For this review, take the finished solid that the model builds, in its own axes (mm). Face numbers are marked on the shaded views. A direction names the side the tool comes from. Coordinates: 2 decimals unless noted, no trailing zeros. Order: outer loops, then holes, each group sorted by start corner. A loop starts at its lowest first (then second) coordinate and runs counter-clockwise, first axis right, second up.
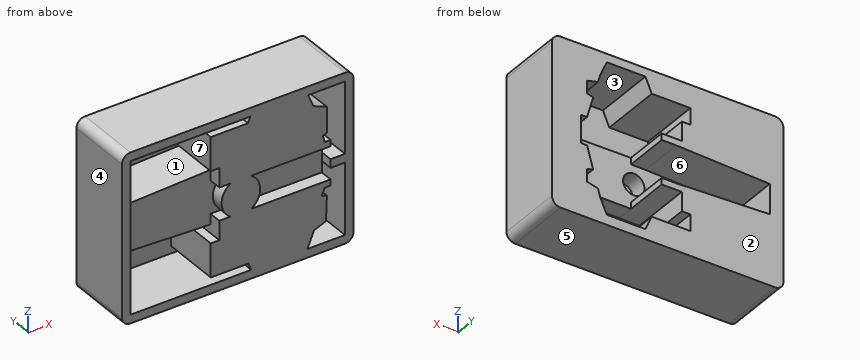
from build123d import *

# Parameters (mm, degrees)
SKETCH1_W                = 54
SKETCH1_H                = 39.25
BOSS_EXTRUDE1_DEPTH      = 15.5
FILLET1_R                = 2
FILLET2_R                = 2
E_WING_START             = 8.464149768
E_WING_BLANK_DEPTH       = 10.5
E_WING_START_2           = 4.464149768
E_WING_BLANK_2_OUTLINE_R = 2.5
E_WING_BLANK_2_DEPTH     = 4
BODY_MOVE_COPY5_ANGLE    = 90
CUT_EXTRUDE1_DEPTH       = 13.5
CUT_EXTRUDE2_DEPTH       = 3


with BuildPart() as part:
    # Sketch1 → Boss-Extrude1 (new body)
    with BuildSketch(Plane(origin=(0, 0, 0), x_dir=(1, 0, 0), z_dir=(0, 1, 0))):
        with Locations((27, 19.625)):
            Rectangle(SKETCH1_W, SKETCH1_H)
    extrude(amount=BOSS_EXTRUDE1_DEPTH)

    # Fillet1
    fillet1_edges = [part.edges().sort_by_distance(p)[0] for p in [
        (0, 7.75, 0),
    ]]
    fillet(fillet1_edges, radius=FILLET1_R)

    # Fillet2
    fillet2_edges = [part.edges().sort_by_distance(p)[0] for p in [
        (0, 7.75, -39.25),
        (54, 7.75, -39.25),
        (54, 7.75, 0),
    ]]
    fillet(fillet2_edges, radius=FILLET2_R)


with BuildPart() as body_2:
    # E-Wing Blank: read off the stored shape, not the designer's step
    # E-Wing Blank outline → E-Wing Blank (new body)
    with BuildSketch(Plane(origin=(0, 0, 0), x_dir=(1, 0, 0), z_dir=(0, 1, 0)).offset(E_WING_START)):
        Polygon((76.333039674, 32.997673143), (76.333039674, 31.604556958), (82.819483769, 31.604556958), (82.819483769, 32.997673143), (87.846693693, 34.426348928), (88.252707074, 32.997673143), (91.160450403, 32.997673143), (91.794809137, 35.548358356), (93.685930379, 36.085793467), (97.076261721, 37.607956728), (97.076261721, 46.607956728), (93.685930379, 48.085793467), (93.685930379, 57.085793467), (89.860941172, 57.085793467), (89.860941172, 55.085793467), (85.427430955, 55.085793467), (85.427430955, 50.394400823), (83.927430955, 50.394400823), (83.927430955, 53.784732166), (83.058115227, 75.604556958), (76.094408216, 75.604556958), (75.225092487, 53.784732166), (75.225092487, 50.394400823), (73.725092487, 50.394400823), (73.725092487, 55.085793467), (69.29158227, 55.085793467), (69.29158227, 57.085793467), (65.466593064, 57.085793467), (65.466593064, 48.085793467), (62.076261721, 46.607956728), (62.076261721, 37.607956728), (65.466593064, 36.085793467), (67.357714306, 35.548358356), (67.99207304, 32.997673143), (70.899816369, 32.997673143), (71.30582975, 34.426348928), align=None)
    extrude(amount=E_WING_BLANK_DEPTH)

    # E-Wing Blank 2 outline → E-Wing Blank 2 (add)
    with BuildSketch(Plane(origin=(0, 0, 0), x_dir=(1, 0, 0), z_dir=(0, 1, 0)).offset(E_WING_START_2)):
        Polygon((71.30582975, 34.426348928), (73.819434712, 33.712011036), (73.725092487, 50.394400823), (73.725092487, 55.085793467), (69.29158227, 55.085793467), (69.29158227, 57.085793467), (65.466593064, 57.085793467), (65.466593064, 48.085793467), (62.076261721, 46.607956728), (62.076261721, 37.607956728), (65.466593064, 36.085793467), (67.357714306, 35.548358356), (67.99207304, 32.997673143), (70.899816369, 32.997673143), align=None)
        Polygon((85.427430955, 50.394400823), (85.333088731, 33.712011036), (87.846693693, 34.426348928), (88.252707074, 32.997673143), (91.160450403, 32.997673143), (91.794809137, 35.548358356), (93.685930379, 36.085793467), (97.076261721, 37.607956728), (97.076261721, 46.607956728), (93.685930379, 48.085793467), (93.685930379, 57.085793467), (89.860941172, 57.085793467), (89.860941172, 55.085793467), (85.427430955, 55.085793467), align=None)
        with Locations((79.576261721, 51.054553675)):
            Circle(E_WING_BLANK_2_OUTLINE_R)
    extrude(amount=E_WING_BLANK_2_DEPTH)


with BuildPart() as body_2_1:
    # Body-Move/Copy3: moved
    add(body_2.part.moved(Location((0, -2.941364734, 30.286723837))))


with BuildPart() as body_2_2:
    # Body-Move/Copy4: moved
    add(body_2_1.part.moved(Location((-54.380009777, 0, 0))))


with BuildPart() as body_2_3:
    # Body-Move/Copy5: moved
    add(body_2_2.part.rotate(Axis((25.196251944, 0, -23.317833121), (0, 1, 0)), BODY_MOVE_COPY5_ANGLE))


with BuildPart() as body_2_4:
    # Body-Move/Copy6: moved
    add(body_2_3.part.moved(Location((0, 0, 3.871475448))))


with BuildPart() as body_2_5:
    # Body-Move/Copy8: moved
    add(body_2_4.part.moved(Location((0, -0.52, 0))))


with BuildPart() as part_1:
    add(part.part)

    # Intersect1: read off the stored shape, not the designer's step
    # Intersect1: cut body 2
    add(body_2_5.part, mode=Mode.SUBTRACT)

    # Sketch3 → Cut-Extrude1 (cut)
    with BuildSketch(Plane(origin=(0, 0, 0), x_dir=(-1, 0, 0), z_dir=(0, -1, 0))):
        Polygon((-2, 2), (-2, 14.010576961), (-22.715015436, 13.185277541), (-22.715015436, 11.161678222), (-20.715015436, 11.161678222), (-20.715015436, 3.336689015), (-29.405061858, 3.336689015), (-29.944686746, 2), align=None)
        Polygon((-2, 24.882138385), (-22.715015436, 25.707437805), (-22.715015436, 27.731037124), (-20.715015436, 27.731037124), (-20.715015436, 35.556026331), (-29.477301308, 35.556026331), (-30.143460637, 37.25), (-2, 37.25), align=None)
        Polygon((-43.248853496, 37.25), (-44.797063028, 33.545989344), (-47.572936951, 32.454370068), (-47.80313576, 26.676379962), (-46.622265015, 26.276395033), (-47.270268456, 24.671244676), (-48.650700904, 24.671244676), (-48.650700904, 20.614103613), (-52, 20.614103613), (-52, 37.25), align=None)
        Polygon((-48.650700904, 14.203135625), (-47.31395374, 14.203135625), (-47.2997118, 14.169991759), (-46.845009369, 12.553018905), (-47.80313576, 12.280730301), (-47.80313576, 6.298647203), (-44.698842535, 5.001108722), (-43.40926424, 2), (-52, 2), (-52, 18.620885492), (-48.650700904, 18.620885492), align=None)
    extrude(amount=-CUT_EXTRUDE1_DEPTH, mode=Mode.SUBTRACT)

    # Sketch4 → Cut-Extrude2 (cut)
    with BuildSketch(Plane.XZ):
        with BuildLine():
            Line((2, -14.010576961), (2, -24.882138385))
            Line((2, -24.882138385), (22.715015436, -25.707437805))
            Line((22.715015436, -25.707437805), (22.715015436, -23.250355795))
            Line((22.715015436, -23.250355795), (25.342175719, -23.250355795))
            ThreePointArc((25.342175719, -23.250355795), (23.246255228, -19.446357673), (25.342175719, -15.642359551))
            Line((25.342175719, -15.642359551), (22.715015436, -15.642359551))
            Line((22.715015436, -15.642359551), (22.715015436, -13.185277541))
            Line((22.715015436, -13.185277541), (2, -14.010576961))
        make_face()
        with BuildLine():
            Line((48.650700904, -23.250355795), (48.650700904, -20.614103613))
            Line((48.650700904, -20.614103613), (48.650700904, -18.620885492))
            Line((48.650700904, -18.620885492), (48.650700904, -15.642359551))
            Line((48.650700904, -15.642359551), (30.150334738, -15.642359551))
            ThreePointArc((30.150334738, -15.642359551), (32.246255228, -19.446357673), (30.150334738, -23.250355795))
            Line((30.150334738, -23.250355795), (48.650700904, -23.250355795))
        make_face()
    extrude(amount=-CUT_EXTRUDE2_DEPTH, mode=Mode.SUBTRACT)


solid = part_1.part
1. Take a section at B-B, the plane y = 6.5. Give the number of separate pieces and of enclosed holes in the cut face, plus the area to 3 significant figures.
Answer below:
separate pieces: 1
enclosed holes: 5
area: 629 mm2
2. Take a section at C-C, the plane z = -29. Give the boundary of the cut face in (x, y).
Answer below:
outline: (0, 0) - (2, 0) - (2, 13.5) - (20.72, 13.5) - (20.72, 0) - (47.71, 0) - (47.71, 13.5) - (52, 13.5) - (52, 0) - (54, 0) - (54, 15.5) - (45.8, 15.5) - (45.8, 1) - (23.72, 1) - (23.72, 15.5) - (0, 15.5) - close
3. The part is to be moulded in two halves that separate along X. For the marked faces 4, 5, 6 and 7, say which applies: +X half, -X half, draft (parallel to the pull), parting line (faces both ways), or undercut.
Answer below:
face 4: -X half
face 5: draft
face 6: undercut
face 7: undercut
4. To check wall thickness, follow L1, parallel to Z at x = 51, y = 10.25; L2, parallel to X at y = 13, z = -17; L3, parallel to X at y = 10.75, z = -9. State the ranges of each line that lie inside material, in increasing order.
Answer below:
L1: z = -39.25 to -37.25, -20.61 to -18.62, -2 to 0
L2: x = 0 to 3.2, 47.2 to 48.65, 52 to 54
L3: x = 0 to 2, 20.72 to 21.72, 45.8 to 47.8, 52 to 54
5. Take a section at A-A, the plane x = 17.5. Give the boundary of the cut face in (y, z), plus the area to 3 significant figures.
Answer below:
outline: (0, -39.25) - (15.5, -39.25) - (15.5, -23.5) - (5, -23.5) - (5, -15.39) - (15.5, -15.39) - (15.5, 0) - (0, 0) - (0, -2) - (13.5, -2) - (13.5, -13.39) - (3, -13.39) - (3, -25.5) - (13.5, -25.5) - (13.5, -37.25) - (0, -37.25) - close
area: 175 mm2
6. Machinability: for the marked faces 1, 2 and 3, which of the approach directions +Z, -Z, +X, -X, +Y, -Y give a long, thin tool a straight path to every point of the face, cutting with its end or side? Answer none if there is none.
Answer below:
face 1: -Y
face 2: +Z, -Z, +X, -X, +Y
face 3: +Y
7. Take a section at D-D, the plane x = 26.5. Give the boundary of the cut face in (y, z), plus the area to 3 significant figures.
Answer below:
outline: (0, -39.25) - (15.5, -39.25) - (15.5, -33.56) - (1, -33.56) - (1, -25.3) - (15.5, -25.3) - (15.5, -23.8) - (5, -23.8) - (5, -21.61) - (1, -21.61) - (1, -17.28) - (5, -17.28) - (5, -15.1) - (15.5, -15.1) - (15.5, -13.6) - (1, -13.6) - (1, -5.34) - (15.5, -5.34) - (15.5, 0) - (0, 0) - (0, -2) - (13.5, -2) - (13.5, -3.34) - (0, -3.34) - (0, -35.56) - (13.5, -35.56) - (13.5, -37.25) - (0, -37.25) - close
area: 219 mm2
8. Clearance check with flat-ended pins moving along their axes: pin 1 Ø4 at (x, z) = (36, -4.5) entering from +Y; pin 2 Ø4 at (x, z) = (12.5, -22.5) entering from -Y. State where each tip first meets the part, or that it passes through.
Answer below:
pin 1: stops at y = 1
pin 2: stops at y = 3
